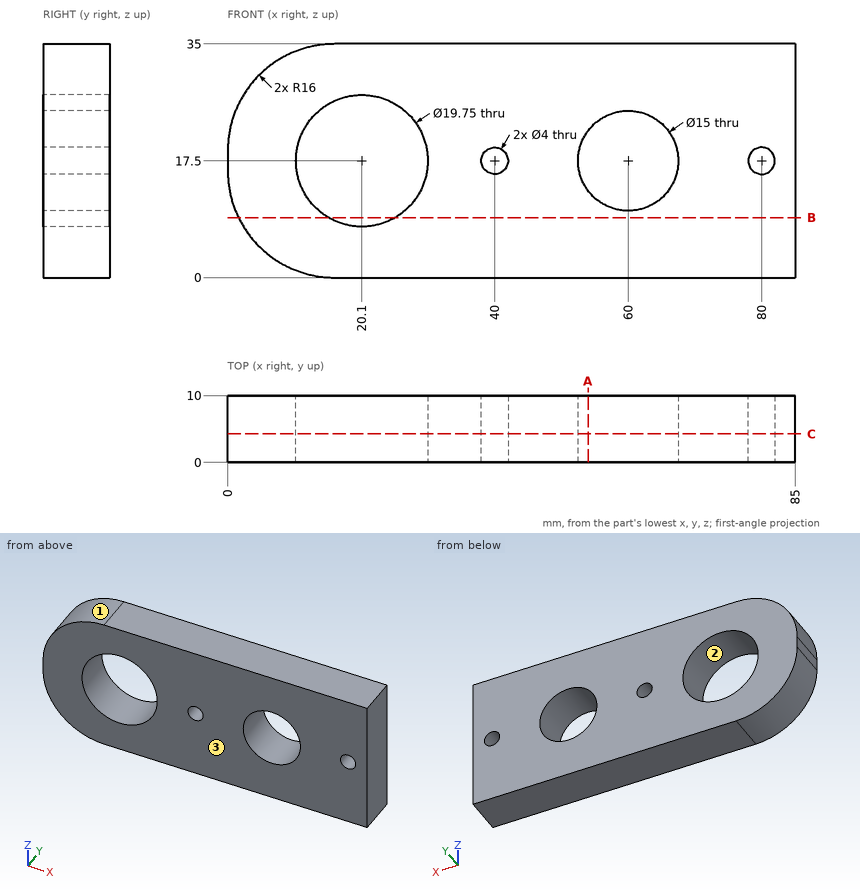
For this review, use the dimensioned drawing (mm, ordinates from the lowest corner) and the shaded views. Give positions to 0.01 mm unless a question says otherwise; leave off trailing zeros. Write each loop counter-clockwise with the first axis right and the second up, starting at its lowest first coordinate (ties: lowest second). Pieces come first, ordered by that corner, then holes. Notation, with made-up numbers: M 88.5,41.5 L 114.5,41.5 A28 ccw 114.5,67.5 Z; hole C 4.25,13 d6. An arc over 180 degrees is marked long. Answer as a JSON object with one key per item and string values. Group by question number.
Item 1: Draft analysis for pull direction X (two halves, no side actions). For the marked faces 1, 2 and 3, state which applies: +X half, -X half, draft (parallel to the pull), parting line (faces both ways), or undercut.
Item 2: Consider section A-A on x = 54. Write out the cut boundary in (y, z), plus the area to 3 significant figures.
Item 3: Consider section C-C on y = 4.25. Write out the cut boundary in (x, z) (3 decimals), plus the area to 3 significant figures.
Item 4: For probe 1 along Z at (x, y) = (80, 6.25); probe 2 along X at (y, z) = (1.25, 16.5); probe 3 along Z at (x, y) = (20.1, 7.5) (3 decimals), list the stretches that pass through material, from the lowest coordinate up. Write a range as [from, to].
Item 5: For pin 1 Ø12 at (x, z) = (60, 17.5) entering from +Y; pin 2 Ø4 at (x, y) = (11.5, 8) entering from +Z, all flat-tipped, find the tip position at first contact; note any pin that passes through.
Item 6: Consider section B-B on z = 9. Write out the cut boundary in (x, y).
Check result:
{
 "1": {"face 1": "-X half", "face 2": "undercut", "face 3": "draft"},
 "2": {"outline": "M 0,0 L 10,0 L 10,13 L 0,13 Z; M 0,22 L 10,22 L 10,35 L 0,35 Z", "area": "260 mm^2"},
 "3": {"outline": "M 0,16 A16 ccw 16,0 L 85,0 L 85,35 L 16,35 A16 ccw 0,19 Z; hole C 20.1,17.5 d19.75; hole C 40,17.5 d4; hole C 60,17.5 d15; hole C 80,17.5 d4", "area": "2,360 mm^2"},
 "4": {"probe 1": "z = [0, 15.5], [19.5, 35]", "probe 2": "x = [0, 10.28], [29.92, 38.27], [41.73, 52.57], [67.43, 78.27], [81.73, 85]", "probe 3": "z = [0, 7.625], [27.375, 35]"},
 "5": {"pin 1": "passes through", "pin 2": "stops at z = 34.8"},
 "6": {"outline": "M 1.61,0 L 15.07,0 L 15.07,10 L 1.61,10 Z; M 25.13,0 L 85,0 L 85,10 L 25.13,10 Z"}
}
